CAD build for the part. Positions are in the model's coordinates, mm. A direction names the side the tool comes from. Round coordinates to 2 decimals unless told otherwise and drop trailing zeros. Loops run counter-clockwise (first coordinate to the right, second up) from the corner with the lowest first, then second, coordinate; pieces in that order, holes last. Notation, with made-up numbers: (53.5, -4.75) - (76.5, -4.75) arc R8 ccw to (76.5, -0.75) - close; hole circle Ø1 at (89.5, 36). An arc over 180 degrees is marked (long way). Use one line per item in the form item = value.
from build123d import *

# Parameters (mm, degrees)
SKETCH_3_R               = 7.25
CUT_EXTRUDE_1_DEPTH      = 12
CUT_EXTRUDE_3_DEPTH      = 39.897300678
CUT_EXTRUDE_2_DEPTH      = 16
CUT_EXTRUDE_2_DEPTH_BACK = 10
SKETCH_4_R               = 2.1
M2X0_41_D                = 1.6
M2X0_41_DEPTH            = 7
M2X0_41_CSINK_D          = 2.2
M2X0_41_CSINK_ANGLE      = 90
M2X0_41_TIP              = 0.480688495
SKETCH_12_R              = 7.25
SKETCH_12_R_2            = 5.25
CUT_EXTRUDE_4_DEPTH      = 0.8


# Read off the part's stored shape, not the designer's step: Отверстие обработанное метчиком M3x0.51
with BuildPart() as part:
    # Эскиз2 → Повернуть1 (revolve)
    with BuildSketch(Plane.XY, mode=Mode.PRIVATE) as revolve_1_sk:
        Polygon((0, 10), (5, 10), (5, 24), (19, 24), (19, 7.25), (12.1, 7.25), (12.1, 2.5), (6.9, 2.5), (6.9, 7.25), (0, 7.25), align=None)
    revolve(revolve_1_sk.sketch.rotate(Axis((0, 0, 0), (1, 0, 0)), 90), axis=Axis((0, 0, 0), (1, 0, 0)))

    # Эскиз3 → Вырез-Вытянуть1 (cut)
    with BuildSketch(Plane(origin=(19, 0, 0), x_dir=(0, 0, -1), z_dir=(1, 0, 0))):
        with Locations((0, -15)):
            Circle(SKETCH_3_R)
    extrude(amount=-CUT_EXTRUDE_1_DEPTH, mode=Mode.SUBTRACT)

    # Эскиз5 → Вырез-Вытянуть3 (cut, through all)
    with BuildSketch(Plane(origin=(19, 0, 0), x_dir=(0, 0, -1), z_dir=(1, 0, 0))):
        with BuildLine():
            ThreePointArc((24, 0), (-13.638181697, 19.748417658), (-8.5, -22.444375687))
            Line((-8.5, -22.444375687), (-8.5, 8))
            Line((-8.5, 8), (8.5, 8))
            Line((8.5, 8), (8.5, -22.444375687))
            ThreePointArc((8.5, -22.444375687), (19.748417658, -13.638181697), (24, 0))
        make_face()
    extrude(amount=-CUT_EXTRUDE_3_DEPTH, mode=Mode.SUBTRACT)

    # Эскиз4 → Вырез-Вытянуть2 (cut, two sides: drawn at the far end of the back side and taken through both)
    with BuildSketch(Plane(origin=(0, 0, 0), x_dir=(1, 0, 0), z_dir=(0, 1, 0)).offset(-CUT_EXTRUDE_2_DEPTH_BACK)):
        with Locations(Location((9.5, 0, 0), (0, 0, 90))):
            Circle(SKETCH_4_R)
    extrude(amount=CUT_EXTRUDE_2_DEPTH + CUT_EXTRUDE_2_DEPTH_BACK, mode=Mode.SUBTRACT)

    # Отверстие обработанное метчиком M3x0.51 outline → Отверстие обработанное метчиком M3x0.51 (revolve, cut)
    with BuildSketch(Plane(origin=(9.5, 4, 0), x_dir=(1, 0, 0), z_dir=(0, -1, 0))):
        Polygon((1.25, -8.1), (1.25, -1.687245944), (0, -1.687245944), (0, -8.5), (1.65, -8.5), align=None)
    revolve(axis=Axis((9.5, 4, 0), (0, 0, 1)), mode=Mode.SUBTRACT)

    # Отверстие обработанное метчиком M2x0.41
    with Locations(Plane(origin=(19, 0, 0), x_dir=(0, 0, -1), z_dir=(1, 0, 0))):
        with Locations((-6.5, 6.5), (6.5, 6.5), (6.5, -6.5), (-6.5, -6.5), (-6.5, -21), (6.5, -21)):
            CounterSinkHole(M2X0_41_D / 2, M2X0_41_CSINK_D / 2, depth=M2X0_41_DEPTH, counter_sink_angle=M2X0_41_CSINK_ANGLE)
            with Locations((0, 0, -(M2X0_41_DEPTH + M2X0_41_TIP / 2))):  # 118° drill point
                Cone(0, M2X0_41_D / 2, M2X0_41_TIP, mode=Mode.SUBTRACT)

    # Эскиз12 → Вырез-Вытянуть4 (cut)
    with BuildSketch(Plane(origin=(7, 0, 0), x_dir=(0, 0, -1), z_dir=(1, 0, 0))):
        with Locations((0, -15)):
            Circle(SKETCH_12_R)
        with Locations((0, -15)):
            Circle(SKETCH_12_R_2, mode=Mode.SUBTRACT)
    extrude(amount=-CUT_EXTRUDE_4_DEPTH, mode=Mode.SUBTRACT)

    # Эскиз13 → Отверстие обработанное метчиком M6x0.51 (revolve, cut)
    with BuildSketch(Plane(origin=(7, -15, 0), x_dir=(0, 0, -1), z_dir=(0, 1, 0))):
        Polygon((0, 0), (0, 2), (3.1, 2), (2.75, 1.65), (2.75, 0.35), (3.1, 0), align=None)
    revolve(axis=Axis((13.35, -15, 0), (-1, 0, 0)), mode=Mode.SUBTRACT)


solid = part.part
1) Tool access for faces 4 (the cylindrical face through (6.606, -9.795, 0.683)), 5 (the flat face through (5, 7, 8)), 6 (the flat face through (19, -8, -4)): list every direction of +Z, -Z, +X, -X, +Y, -Y with a clear straight run to the whole face (end or side of a thin tool).
Report:
face_4 = +X
face_5 = +Z, -X, +Y
face_6 = +Z, -Z, +X, +Y, -Y
2) Slice it at D-D (y = -9). Write the cut outline in (x, z).
Report:
outline = (0, -4.36) - (5, -4.36) - (5, -8.5) - (19, -8.5) - (19, -4.07) - (6.2, -4.07) - (6.2, 4.07) - (19, 4.07) - (19, 8.5) - (5, 8.5) - (5, 4.36) - (0, 4.36) - close
3) Slice it at A-A (x = 16.75). State how many separate pieces and enclosed holes the cut face has, plus the area to 3 significant figures.
Report:
separate_pieces = 1
enclosed_holes = 8
area = 193 mm^2
4) Two-plate mould, pull along Y, no slides. Class faces 1 (the cylindrical face through (8.869, -4.759, -2.003)), 2 (the cylindrical face through (3.4, 6.43, 3.35)), 3 (the cylindrical face through (2.535, 6.731, -7.395)): +Y half, -Y half, draft (parallel to the pull), parting line (faces both ways), or undercut.
Report:
face_1 = draft
face_2 = undercut
face_3 = +Y half
5) Slice it at B-B (y = 0). Write the cut outline in (x, z), plus the area to 3 significant figures.
Report:
outline = (0, -8.5) - (19, -8.5) - (19, -7.25) - (12.1, -7.25) - (12.1, -2.5) - (6.9, -2.5) - (6.9, -7.25) - (0, -7.25) - close; (0, 7.25) - (6.9, 7.25) - (6.9, 2.5) - (12.1, 2.5) - (12.1, 7.25) - (19, 7.25) - (19, 8.5) - (0, 8.5) - close
area = 96.9 mm^2
6) Drill centre lines: probe 1 along X at (y, z) = (-4.5, 0); probe 2 along X at (y, z) = (4, -5); probe 3 along Z at (x, y) = (15.75, -21). Where is each one in solid material? Low to high.
Report:
probe_1 = 6.9 to 7.4, 11.6 to 12.1
probe_2 = 6.9 to 8.25, 10.75 to 12.1
probe_3 = -8.5 to -7.3, -5.7 to -4.07, 4.07 to 5.7, 7.3 to 8.5
7) Flat gauge pins, fed straight in: pin 1 (4.5 mm diameter, centred on y = -17, z = -1, fed in from +X); pin 2 (2 mm diameter, centred on x = 9.5, y = 4, fed in from -Z); pin 3 (2 mm diameter, centred on x = 9, z = 1.5, fed in from -Y). Where does each tip first touch, or does it go through?
Report:
pin_1 = 7
pin_2 = 1.85
pin_3 = -23.99
